Autodesk Inventor part; units mm, degrees
ref_plane "YZ Plane" through (0, 0, 0) normal (1, 0, 0) x (0, 1, 0)
ref_plane "XZ Plane" through (0, 0, 0) normal (0, 1, 0) x (-1, 0, 0)
ref_plane "XY Plane" through (0, 0, 0) normal (0, 0, 1) x (1, 0, 0)
sketch "Náčrt1" plane through (0, 0, 0) normal (0, 0, 1) x (1, 0, 0)
  line L0 (0, 0) -> (110, 0)
  line L1 (110, 0) -> (110, 72.5558)
  line L2 (67.945, 110) -> (0, 110)
  line L3 (0, 110) -> (0, 0)
  line L4 (0, 0) -> (268.4899, 0) construction
  line L5 (166.1231, 136.1347) -> (115.2721, 85.2837)
  line L6 (135.1648, 167.093) -> (80.3503, 114.9574)
  line L7 (166.1231, 136.1347) -> (135.1648, 167.093)
  arc A0 (115.2721, 85.2837) -> (110, 72.5558) centre (128, 72.5558) ccw
  arc A1 (67.945, 110) -> (80.3503, 114.9574) centre (67.945, 128) ccw
extrude "Vysunutí1" add sketch "Náčrt1" along normal blind 10
sketch "Náčrt2" plane through (0, 0, 10) normal (0, 0, 1) x (1, 0, 0)
  line L0 (0, 0) -> (110, 0)
  line L1 (0, 0) -> (5, 0) construction
  line L2 (3.5355, 3.5355) -> (13.5355, 3.5355)
  line L3 (8.5355, 28.5355) -> (3.5355, 28.5355)
  line L4 (3.5355, 28.5355) -> (3.5355, 3.5355)
  line L5 (3.5355, 3.5355) -> (28.5355, 3.5355)
  line L6 (28.5355, 3.5355) -> (28.5355, 8.5355)
  line L7 (3.5355, 13.5355) -> (3.5355, 3.5355)
  line L8 (13.5355, 28.5355) -> (8.5355, 28.5355)
  line L9 (8.5355, 28.5355) -> (8.5355, 13.5355)
  line L10 (13.5355, 13.5355) -> (13.5355, 18.5355)
  line L11 (28.5355, 13.5355) -> (13.5355, 13.5355)
  line L12 (8.5355, 13.5355) -> (8.5355, 8.5355)
  line L13 (8.5355, 8.5355) -> (28.5355, 8.5355)
  line L14 (28.5355, 8.5355) -> (28.5355, 13.5355)
  line L15 (13.5355, 28.5355) -> (13.5355, 18.5355)
  line L16 (13.5355, 18.5355) -> (8.5355, 18.5355)
extrude "Vysunutí2" add sketch "Náčrt2" along normal blind 5 contours L4 L3 L9 L12 L13 L6 L5 L2
extrude "Vysunutí3" add sketch "Náčrt2" along normal blind 10 contours L13 L12 L9 L16 L10 L11 L14 | L8 L15 L16 L9
sketch "Náčrt5" plane through (13.5355, 13.5355, 10) normal (1, 0, 0) x (0, 0, -1)
  line L0 (-5, -5) -> (-5, 15)
  line L1 (-10, 15) -> (-5, 15)
  line L2 (-5, 15) -> (-5, 5)
  line L3 (-5, 5) -> (-10, 5)
  line L4 (-10, 5) -> (-10, 15)
  point P0 (10, -13.5355)
extrude "Vysunutí4" add sketch "Náčrt5" along normal blind 2
sketch "Náčrt7" plane through (13.5355, 13.5355, 10) normal (0, 1, 0) x (1, 0, 0)
  line L0 (15, -10) -> (0, -10)
  line L1 (15, -5) -> (-5, -5)
  line L2 (15, -10) -> (5, -10)
  line L3 (5, -10) -> (5, -5)
  line L4 (5, -5) -> (15, -5)
  line L5 (15, -5) -> (15, -10)
  point P0 (-13.5355, 10)
extrude "Vysunutí5" add sketch "Náčrt7" along normal blind 2
sketch "Náčrt8" plane through (0, 0, 10) normal (0, 0, 1) x (1, 0, 0)
  line L0 (0, 110) -> (0, 0)
  line L1 (0, 110) -> (10, 110) construction
  circle A0 centre (7.0711, 102.9289) radius 2.5
extrude "Vysunutí6" cut sketch "Náčrt8" against normal blind 20
sketch "Náčrt9" plane through (0, 0, 10) normal (0, 0, 1) x (1, 0, 0)
  line L0 (0, 0) -> (110, 0)
  line L1 (110, 0) -> (102.9289, 7.0711)
  line L2 (110, 0) -> (120, 0) construction
  circle A0 centre (102.9289, 7.0711) radius 2.5
  dimension "d36" = 5
extrude "Vysunutí7" cut sketch "Náčrt9" against normal blind 20
sketch "Náčrt13" plane through (135.1648, 167.093, 0) normal (0.7071, 0.7071, 0) x (-0.7071, 0.7071, 0)
  line L0 (-22.5767, 0) -> (-22.5767, 10)
  line L1 (-22.5767, 15) -> (-22.5767, 20)
  line L2 (-22.5767, 20) -> (-36.7188, 20)
  line L3 (55.2051, 10) -> (-22.5767, 10)
  circle A0 centre (-22.5767, 20) radius 10
  dimension "d43" = 10
extrude "Vysunutí8" add sketch "Náčrt13" against normal blind 50
sketch "Náčrt14" plane through (151.1289, 151.1289, 20) normal (0.7071, 0.7071, 0) x (-0.7071, 0.7071, 0)
  line L0 (0, 0) -> (-14.1421, 0)
  circle A0 centre (0, 0) radius 5
  line L1 (0, -5) -> (14.1421, -5)
  point P0 (0, -20)
extrude "Vysunutí9" cut sketch "Náčrt14" against normal blind 50
sketch "Náčrt15" plane through (0, 0, 10) normal (0, 0, 1) x (1, 0, 0)
  line L0 (108.7025, 122.8446) -> (122.8446, 108.7025)
  line L1 (122.8446, 108.7025) -> (126.3801, 105.1669)
  line L2 (115.2721, 85.2837) -> (166.1231, 136.1347)
  line L3 (126.3801, 105.1669) -> (129.9157, 108.7025)
  line L4 (129.9157, 108.7025) -> (108.7025, 129.9157)
  line L5 (112.238, 126.3801) -> (108.7025, 129.9157)
  line L6 (105.1669, 126.3801) -> (108.7025, 129.9157)
  line L7 (105.1669, 126.3801) -> (122.8446, 108.7025)
  point P0 (0, 0)
  point P1 (115.7735, 115.7735)
  dimension "d48" = 5
extrude "Vysunutí10" add sketch "Náčrt15" along normal blind 4.5
sketch "Náčrt16" plane through (0, 0, 10) normal (0, 0, 1) x (1, 0, 0)
  line L0 (119.3091, 119.3091) -> (129.9157, 108.7025)
  line L1 (151.1289, 136.9867) -> (154.6644, 133.4512)
  line L2 (154.6644, 133.4512) -> (151.1289, 129.9157)
  line L3 (151.1289, 129.9157) -> (133.4512, 147.5933)
  line L4 (135.1648, 167.093) -> (80.3503, 114.9574)
  line L5 (133.4512, 154.6644) -> (151.1289, 136.9867)
  line L6 (144.0578, 158.1999) -> (108.7025, 122.8446)
  line L7 (133.4512, 147.5933) -> (129.9157, 151.1289)
  line L8 (129.9157, 151.1289) -> (133.4512, 154.6644)
  point P0 (0, 0)
extrude "Vysunutí11" add sketch "Náčrt16" along normal blind 4.5
sketch "Náčrt17" plane through (0, 0, 14.5) normal (0, 0, 1) x (1, 0, 0)
  line L0 (108.7025, 129.9157) -> (105.1669, 126.3801)
  circle A0 centre (108.7025, 126.3801) radius 1.25
  point P0 (0, 0)
extrude "Vysunutí12" add sketch "Náčrt17" along normal blind 1
sketch "Náčrt18" plane through (0, 0, 14.5) normal (0, 0, 1) x (1, 0, 0)
  line L0 (140.5223, 140.5223) -> (129.9157, 151.1289)
  line L1 (129.9157, 151.1289) -> (133.4512, 154.6644)
  circle A0 centre (133.4512, 151.1289) radius 1.25
  point P0 (0, 0)
extrude "Vysunutí13" add sketch "Náčrt18" along normal blind 1
sketch "Náčrt19" plane through (0, 0, 14.5) normal (0, 0, 1) x (1, 0, 0)
  line L0 (154.6644, 133.4512) -> (151.1289, 129.9157)
  circle A0 centre (151.1289, 133.4512) radius 1.25
  point P0 (0, 0)
extrude "Vysunutí14" add sketch "Náčrt19" along normal blind 1
sketch "Náčrt20" plane through (0, 0, 14.5) normal (0, 0, 1) x (1, 0, 0)
  line L0 (119.3091, 119.3091) -> (129.9157, 108.7025)
  line L1 (126.3801, 105.1669) -> (105.1669, 126.3801)
  circle A0 centre (126.3801, 108.7025) radius 1.25
  point P0 (0, 0)
extrude "Vysunutí15" add sketch "Náčrt20" along normal blind 1
sketch "Náčrt22" plane through (0, 0, 15) normal (0, 0, 1) x (1, 0, 0)
  line L0 (18.5355, 13.5355) -> (18.5355, 15.5355)
  line L1 (18.5355, 15.5355) -> (15.5355, 15.5355)
  line L2 (15.5355, 15.5355) -> (95.5355, 15.5355)
  line L3 (95.5355, 15.5355) -> (95.5355, 95.5355)
  line L4 (95.5355, 95.5355) -> (15.5355, 95.5355)
  line L5 (15.5355, 95.5355) -> (15.5355, 15.5355)
  point P0 (0, 0)
  dimension "d63" = 80
  dimension "d64" = 80
extrude "Vysunutí16" add sketch "Náčrt22" along normal blind 7
sketch "Náčrt25" plane through (0, 0, 10) normal (0, 0, 1) x (1, 0, 0)
  line L0 (95.5355, 95.5355) -> (95.5355, 85.5355)
  line L1 (95.5355, 15.5355) -> (95.5355, 95.5355)
  line L2 (15.5355, 95.5355) -> (15.5355, 15.5355)
  line L3 (85.5355, 85.5355) -> (25.5355, 85.5355)
  line L4 (95.5355, 85.5355) -> (85.5355, 85.5355)
  line L5 (85.5355, 85.5355) -> (85.5355, 25.5355)
  line L6 (85.5355, 25.5355) -> (25.5355, 25.5355)
  line L7 (25.5355, 25.5355) -> (25.5355, 85.5355)
  point P0 (0, 0)
extrude "Vysunutí17" add sketch "Náčrt25" along normal blind 5
sketch "Náčrt26" plane through (0, 0, 22) normal (0, 0, 1) x (1, 0, 0)
  line L0 (95.5355, 95.5355) -> (15.5355, 95.5355)
  line L1 (28.5355, 15.5355) -> (95.5355, 15.5355)
  circle A0 centre (55.5355, 82.2055) radius 9
  circle A1 centre (55.5355, 55.5455) radius 9
  circle A2 centre (55.5355, 28.8655) radius 9
  point P0 (0, 0)
extrude "Vysunutí18" cut sketch "Náčrt26" against normal blind 7
sketch "Náčrt29" plane through (0, 0, 10) normal (0, 0, 1) x (1, 0, 0)
  point P0 (0, 0)
properties part number "Součást1"
Geometry check sheet. Reference: the model listing, model coordinates, mm. A direction names the side the tool comes from. Give positions to 0.01 mm unless a question says otherwise; leave off trailing zeros. Loops run counter-clockwise (first coordinate to the right, second up) from the corner with the lowest first, then second, coordinate; pieces in that order, holes last. Notation, with made-up numbers: M -24,0.25 L -15,0.25 A25 ccw -15,37.25 Z; hole C 57,83.5 d9. An arc over 180 degrees is marked long. Write item = value, one per line.
(1) Material ranges on line 1 (Y direction, x = 62, z = 18.25); line 2 (Z direction, x = 60.5, y = 21); line 3 (Z direction, x = 103, y = 117.5), recorded low to high. Write a range as [from, to].
Answer below:
line_1 = [15.54, 22.6], [35.13, 49.28], [61.81, 75.94], [88.47, 95.54]
line_2 = [0, 10], [15, 22]
line_3 = [0, 10]
(2) Tool access check on faces 1 (the face through (95.536, 55, 18)), 2 (the face through (56, 95.536, 18)), 3 (the face through (136.323, 151.792, 11.719)), 4 (the face through (16, 3.536, 12)). Record the directions out of +Z, -Z, +X, -X, +Y, -Y that give a thin tool (end or side, any length) a straight path to the whole face; none if there is none.
Answer below:
face_1 = +Z, +X, +Y, -Y
face_2 = +Z, +X, -X, +Y
face_3 = +Y
face_4 = +Z, +X, -X, -Y
(3) Gauge pin test, flat ends, axial feed: pin 1 Ø4 at (y, z) = (113.5, 24) entering from -X; pin 2 Ø6 at (x, y) = (61.5, 67.5) entering from -Z; pin 3 Ø1 at (y, z) = (105, 12.5) entering from -X; pin 4 Ø4 at (x, y) = (83, 87) entering from +Z. Record the tip position at first contact, or that the pin passes through.
Answer below:
pin_1 = 116.29
pin_2 = 0
pin_3 = 126.05
pin_4 = 22
(4) Release check for a two-part mould opening along X. For faces 5 (the face through (135, 151, 14.5)), 6 (the face through (54, 0, 5)), 7 (the face through (108.14, 141.39, 4.93)) record: released by +X, released by -X, zero draft, split by the parting line, or undercut.
Answer below:
face_5 = undercut
face_6 = zero draft
face_7 = released by -X
(5) Sectioned sample at A-A, the plane x = 22. Record the cut outline in (y, z), plus the area to 4 significant figures.
Answer below:
outline = M 0,0 L 110,0 L 110,10 L 13.54,10 L 13.54,15 L 95.54,15 L 95.54,22 L 15.54,22 L 15.54,20 L 8.54,20 L 8.54,15 L 3.54,15 L 3.54,10 L 0,10 Z
area = 1,745 mm2
(6) Sectioned sample at B-B, the plane x = 75. Record the cut outline in (y, z).
Answer below:
outline = M 0,0 L 111.44,0 L 111.44,10 L 85.54,10 L 85.54,15 L 95.54,15 L 95.54,22 L 15.54,22 L 15.54,15 L 25.54,15 L 25.54,10 L 0,10 Z
